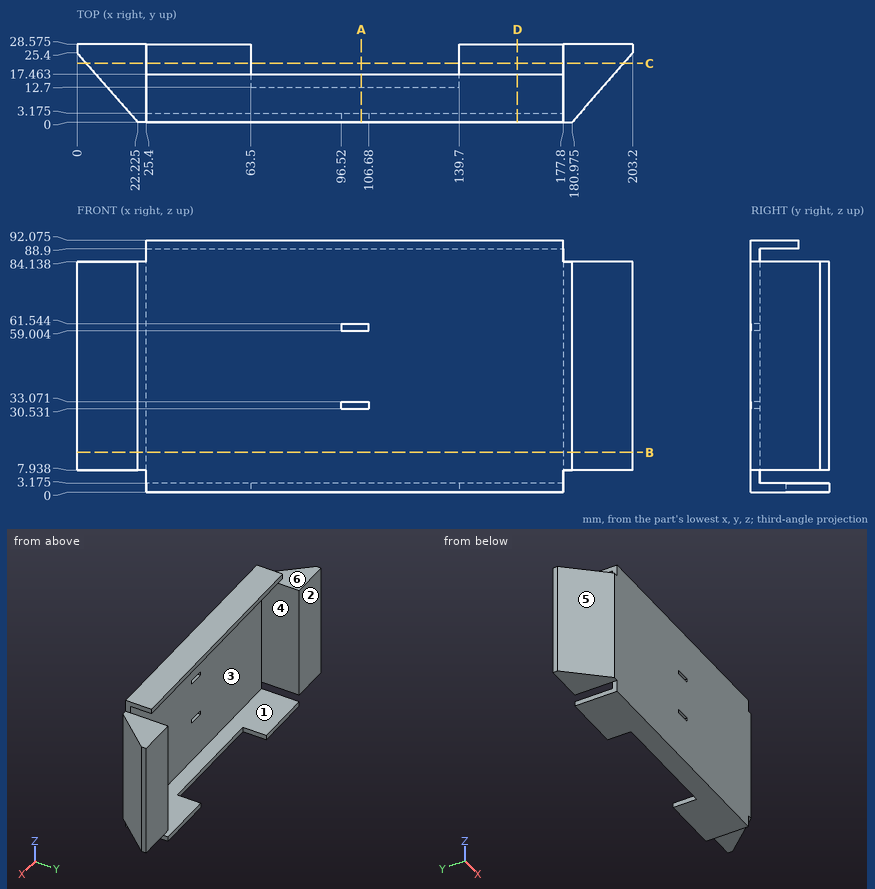
Verification items for this drawing (mm, ordinates from the low corner). A direction names the side the tool comes from. Round coordinates to 2 decimals unless told otherwise and drop trailing zeros. Loops run counter-clockwise (first coordinate to the right, second up) from the corner with the lowest first, then second, coordinate; pieces in that order, holes last. Notation, with made-up numbers: (68, 63) -> (127, 63) arc R21 cw to (127, 81) -> close; hole circle Ø11 at (83.5, 3.25). An arc over 180 degrees is marked (long way). Answer in a Markdown table with one row per item.
Q1. Sectioned sample at A-A on x = 104. Enter the section's corners in (y, z) (1 decimal), then the cut area to 3 significant figures.
Data:
| item | result |
|---|---|
| outline | (0, 0) -> (12.7, 0) -> (12.7, 3.2) -> (3.2, 3.2) -> (3.2, 30.5) -> (0, 30.5) -> close; (0, 33.1) -> (3.2, 33.1) -> (3.2, 59) -> (0, 59) -> close; (0, 61.5) -> (3.2, 61.5) -> (3.2, 88.9) -> (17.5, 88.9) -> (17.5, 92.1) -> (0, 92.1) -> close |
| area | 352 mm^2 |
Q2. Go/stop test with flat-tipped pins: P1, Ø1.6, axis at x = 99.5, y = 2, coming from the -Z side; P2, Ø1, axis at y = 13, z = 73, coming from the -X side; P3, Ø12.5, axis at x = 15, y = 16, coming from the +Z side; P4, Ø2.5, axis at y = 21, z = 1.5, coming from the +X side. Record where each tip stops, or that it passes through.
Data:
| item | result |
|---|---|
| P1 | stops at z = 0 |
| P2 | stops at x = 10.41 |
| P3 | stops at z = 84.14 |
| P4 | stops at x = 177.8 |
Q3. Set-up check for the marked faces 1, 2 and 3: record each of +Z, -Z, +X, -X, +Y, -Y from which the full face is reachable in a straight line by a thin tool's end or side.
Data:
| item | result |
|---|---|
| face 1 | +X, -X, +Y |
| face 2 | +Z, -Z, +X, -X, +Y |
| face 3 | +Y |
Q4. Sectioned sample at D-D on x = 161. Enter the section's corners in (y, z) (1 decimal).
Data:
| item | result |
|---|---|
| outline | (0, 0) -> (28.6, 0) -> (28.6, 3.2) -> (3.2, 3.2) -> (3.2, 88.9) -> (17.5, 88.9) -> (17.5, 92.1) -> (0, 92.1) -> close |
Q5. Thickness scan on L1, parallel to X at y = 27.5, z = 52.5; L2, parallel to Z at x = 51, y = 12.5 (1 decimal); L3, parallel to Y at x = 89, z = 18.5 (1 decimal). Record the ranges inside material, lowest first.
Data:
| item | result |
|---|---|
| L1 | x = 0 to 25.4, 177.8 to 203.2 |
| L2 | z = 0 to 3.2, 88.9 to 92.1 |
| L3 | y = 0 to 3.2 |
Q6. Sectioned sample at B-B on z = 14.5. Enter the section's corners in (x, y) (1 decimal), then the cut area to 3 significant figures.
Data:
| item | result |
|---|---|
| outline | (0, 25.4) -> (22.2, 0) -> (181, 0) -> (203.2, 25.4) -> (203.2, 28.6) -> (177.8, 28.6) -> (177.8, 3.2) -> (25.4, 3.2) -> (25.4, 28.6) -> (0, 28.6) -> close |
| area | 1,370 mm^2 |
Q7. Release check for a two-part mould opening along X. For the marked faces 4, 5 and 6 record: released by +X, released by -X, zero draft, split by the parting line, or undercut.
Data:
| item | result |
|---|---|
| face 4 | undercut |
| face 5 | released by -X |
| face 6 | zero draft |
Q8. Sectioned sample at C-C on y = 21.5. Enter the section's corners in (x, z) (1 decimal).
Data:
| item | result |
|---|---|
| outline | (3.4, 7.9) -> (25.4, 7.9) -> (25.4, 84.1) -> (3.4, 84.1) -> close; (25.4, 0) -> (63.5, 0) -> (63.5, 3.2) -> (25.4, 3.2) -> close; (139.7, 0) -> (177.8, 0) -> (177.8, 3.2) -> (139.7, 3.2) -> close; (177.8, 7.9) -> (199.8, 7.9) -> (199.8, 84.1) -> (177.8, 84.1) -> close |
